The model under review builds one solid part; all positions refer to its coordinate system, in mm. Face numbers are marked on the shaded views. A direction names the side the tool comes from. Give positions to 0.01 mm unless a question says otherwise; leave off trailing zeros. Order: outer loops, then holes, each group sorted by start corner. A loop starts at its lowest first (then second) coordinate and runs counter-clockwise, first axis right, second up. Notation, with made-up numbers: (-0.5, -10.75) - (48.5, -10.75) arc R32 ccw to (48.5, 28.25) - close; hole circle Ø6 at (-20.5, 10). An arc over 180 degrees is marked (long way). Use CSV: the item, a comma, the result in double quotes. Start each with the question number.
```python
from build123d import *

# Parameters (mm, degrees)
F0_R     = 50
F1_DEPTH = 20
F2_DEPTH = 50
F4_DEPTH = 50


with BuildPart() as f1:
    # F0 (on Front) → F1 (new body)
    with BuildSketch(Plane.XZ):
        Circle(F0_R)
        with BuildLine():
            ThreePointArc((0, -15), (7.071068, -17.928932), (10, -25))
            ThreePointArc((10, -25), (-7.071068, -32.071068), (0, -15))
        make_face(mode=Mode.SUBTRACT)
    extrude(amount=F1_DEPTH)

    # F0 (on Front) → F2 (join)
    with BuildSketch(Plane.XZ):
        with BuildLine():
            ThreePointArc((0, -15), (-7.071068, -32.071068), (10, -25))
            ThreePointArc((10, -25), (7.071068, -17.928932), (0, -15))
        make_face()
    extrude(amount=F2_DEPTH)

    # F3 (on face) → F4 (join)
    with BuildSketch(Plane.XZ):
        with BuildLine():
            ThreePointArc((0, -15), (10.606602, -10.606602), (15, 0))
            ThreePointArc((15, 0), (-10.606602, 10.606602), (0, -15))
        make_face()
    extrude(amount=-F4_DEPTH)


solid = f1.part
```
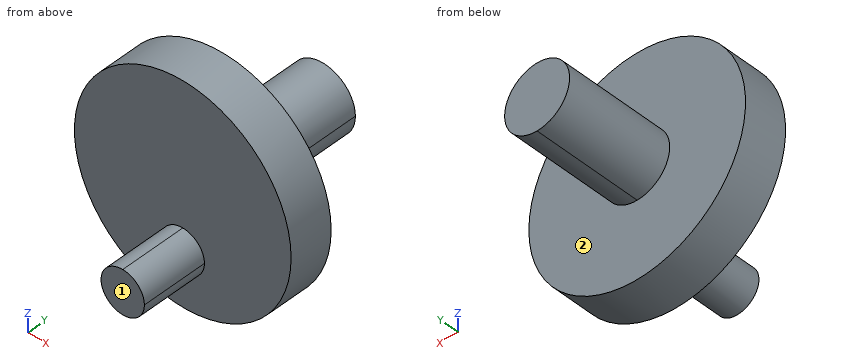
1. Consider section B-B (x = 3.5). Give the boundary of the cut face in (y, z).
2. Consider section A-A (z = -18). Give the boundary of the cut face in (x, y).
3. Consider section D-D (y = 1.5). Give the boundary of the cut face in (x, z).
4. To check wall thickness, follow L1, parallel to Y at x = -25, z = 26.5; L2, parallel to Y at x = -7, z = -12; L3, parallel to X at y = -11, z = 41.5. State the ranges of each line that lie inside material, in increasing order. Write a range as [from, to].
5. Tool access review of the marked faces 1 and 2: name each direction out of +Z, -Z, +X, -X, +Y, -Y from which nothing blocks a thin tool from reaching the whole face with its end or side.
6. Clearance check with flat-ended pins moving along their axes: pin 1 (2 mm diameter, centred on x = -4, y = 35, fed in from -Z); pin 2 (4 mm diameter, centred on y = -7.5, z = -8.5, fed in from -X); pin 3 (1.5 mm diameter, centred on y = 6, z = 4, fed in from -X); pin 4 (8 mm diameter, centred on y = -25, z = 1.5, fed in from -X). State where each tip first meets the part, or that it passes through.
7. Consider section C-C (y = -17). Give the boundary of the cut face in (x, z), and give its area (3 significant figures).
Answers follow:
1,outline,"(-50, -34.37) - (-20, -34.37) - (-20, -49.88) - (0, -49.88) - (0, -14.59) - (50, -14.59) - (50, 14.59) - (0, 14.59) - (0, 49.88) - (-20, 49.88) - (-20, -15.63) - (-50, -15.63) - close"
2,outline,"(-46.65, -20) - (-7.14, -20) - (-7.14, -50) - (7.14, -50) - (7.14, -20) - (46.65, -20) - (46.65, 0) - (-46.65, 0) - close"
3,outline,"(0, -15) arc R15 ccw to (15, 0) arc R15 ccw (long way) to start"
4,L1,"y = [-20, 0]"
4,L2,"y = [-20, 50]"
4,L3,"x = [-27.89, 27.89]"
5,face 1,"+Z, -Z, +X, -X, -Y"
5,face 2,"+Y"
6,pin 1,"stops at z = -14.7"
6,pin 2,"stops at x = -49.58"
6,pin 3,"stops at x = -14.64"
6,pin 4,"passes through"
7,outline,"circle Ø100 at (0, 0)"
7,area,"7,850 mm^2"
